Geometry: final body of the model. Coordinates: model frame, mm. Give positions to 0.01 mm unless a question says otherwise; leave off trailing zeros. Loops run counter-clockwise (first coordinate to the right, second up) from the corner with the lowest first, then second, coordinate; pieces in that order, holes last.
from build123d import *

# Parameters (mm, degrees)
BOSS_EXTRUDE1_DEPTH      = 3
BOSS_EXTRUDE1_DEPTH_BACK = 0.01
FILLET1_R                = 10
FILLET2_R                = 10
FILLET3_R                = 10
FILLET4_R                = 10
CUT_EXTRUDE8_DEPTH       = 10


with BuildPart() as part:
    # Sketch1 → Boss-Extrude1 (new, two sides: drawn at the far end of the back side and taken through both)
    with BuildSketch(Plane.XY.offset(-BOSS_EXTRUDE1_DEPTH_BACK)):
        Polygon((-40, 0), (40, 0), (75, 200), (-75, 200), align=None)
    extrude(amount=BOSS_EXTRUDE1_DEPTH + BOSS_EXTRUDE1_DEPTH_BACK)

    # Fillet1
    fillet1_edges = [part.edges().sort_by_distance(p)[0] for p in [
        (75, 200, 1.495),
    ]]
    fillet(fillet1_edges, radius=FILLET1_R)

    # Fillet2
    fillet2_edges = [part.edges().sort_by_distance(p)[0] for p in [
        (40, 0, 1.495),
    ]]
    fillet(fillet2_edges, radius=FILLET2_R)

    # Fillet3
    fillet3_edges = [part.edges().sort_by_distance(p)[0] for p in [
        (-40, 0, 1.495),
    ]]
    fillet(fillet3_edges, radius=FILLET3_R)

    # Fillet4
    fillet4_edges = [part.edges().sort_by_distance(p)[0] for p in [
        (-75, 200, 1.495),
    ]]
    fillet(fillet4_edges, radius=FILLET4_R)

    # Sketch4 → Cut-Extrude8 (cut)
    with BuildSketch(Plane.XY.offset(3)):
        with BuildLine():
            Line((-1.5, 177), (-1.5, 172.304886114))
            ThreePointArc((-1.5, 172.304886114), (0, 172.75), (1.5, 172.304886114))
            Line((1.5, 172.304886114), (1.5, 177))
            ThreePointArc((1.5, 177), (0, 178.5), (-1.5, 177))
        make_face()
        with BuildLine():
            ThreePointArc((1.5, 170), (0, 168.5), (-1.5, 170))
            Line((-1.5, 170), (-1.5, 172.304886114))
            ThreePointArc((-1.5, 172.304886114), (-1.31101106, 167.582615049), (2.75, 170))
            ThreePointArc((2.75, 170), (2.417384951, 171.31101106), (1.5, 172.304886114))
            Line((1.5, 172.304886114), (1.5, 170))
        make_face()
        with BuildLine():
            Line((-1.5, 172.304886114), (-1.5, 170))
            ThreePointArc((-1.5, 170), (0, 168.5), (1.5, 170))
            Line((1.5, 170), (1.5, 172.304886114))
            ThreePointArc((1.5, 172.304886114), (0, 172.75), (-1.5, 172.304886114))
        make_face()
    extrude(amount=-CUT_EXTRUDE8_DEPTH, mode=Mode.SUBTRACT)


solid = part.part
Item 1: Section query C-C on x = -54. Return loops of the section in (y, z), plus the area to 3 significant figures.
Values follow:
outline: (80, -0.01) - (200, -0.01) - (200, 3) - (80, 3) - close
area: 361 mm2
Item 2: Pin query (flat end, axial travel): pin 1 (1.5 mm diameter, centred on y = 175.5, z = 2, fed in from -X). Return the tip coordinate at first contact, or that it passes through.
Values follow:
pin 1: stops at x = -70.84
Item 3: Ray query, probe 1 along Y at (x, z) = (0, 1.9); probe 2 along X at (y, z) = (170, 2.45); probe 3 along X at (y, z) = (132, 0.4). Return the intervals inside material, ascending.
Values follow:
probe 1: y = 0 to 167.25, 178.5 to 200
probe 2: x = -69.75 to -2.75, 2.75 to 69.75
probe 3: x = -63.1 to 63.1
Item 4: Section query A-A on z = 1.6. Return loops of the section in (x, y), plus the area to 3 significant figures.
Values follow:
outline: (-72.95, 188.28) - (-41.45, 8.28) arc R10 ccw to (-31.6, 0) - (31.6, 0) arc R10 ccw to (41.45, 8.28) - (72.95, 188.28) arc R10 ccw to (63.1, 200) - (-63.1, 200) arc R10 ccw to start; hole (-1.5, 172.3) arc R2.75 ccw (long way) to (1.5, 172.3) - (1.5, 177) arc R1.5 ccw to (-1.5, 177) - close
area: 22,900 mm2
Item 5: Section query B-B on y = 78. Return loops of the section in (x, z), plus the area to 3 significant figures.
Values follow:
outline: (-53.65, -0.01) - (53.65, -0.01) - (53.65, 3) - (-53.65, 3) - close
area: 323 mm2
